Input: dimensioned drawing with shaded views. Units: mm. Origin: part minimum x, y, z. A direction names the side the tool comes from. Round coordinates to 2 decimals unless told otherwise and drop trailing zeros. Loops run counter-clockwise (first coordinate to the right, second up) from the corner with the lowest first, then second, coordinate; pieces in that order, holes last. Notation, with made-up numbers: (68.25, -16.75) - (101.25, -16.75) arc R24 cw to (101.25, 14.25) - close; hole circle Ø11 at (83, -29). An arc over 180 degrees is marked (long way). Answer as a JSON object with one key per item and string values. Group by question number.
Item 1: Line query: line 1 (X direction, y = 1.85, z = 44) (1 decimal); line 2 (Y direction, x = 10, z = 42); line 3 (Z direction, x = 35.5, y = 2.85). Output: solid intervals per line, ascending.
Item 2: Section B-B (y = 1.3). Return the cut outline in (x, z) (1 decimal), plus the area to 3 significant figures.
Item 3: Draft query along Z for the marked faces 1, 2 and 3. Return one class per face: released by +Z, released by -Z, zero draft, split by the parting line, or undercut.
Item 4: First-contact query: pin 1 (1.6 mm diameter, centred on x = 55.48, z = 19.3, fed in from +Y); pin 2 (1 mm diameter, centred on x = 50.5, y = 1.5, fed in from +Z) (1 decimal); pin 3 (1 mm diameter, centred on x = 34.5, y = 2.5, fed in from -Z) (1 decimal); pin 4 (16.5 mm diameter, centred on x = 66, z = 36.5, fed in from +Y). Flat tips, straight axial feed; report the tip coordinate or a pass-through.
Item 5: Reachability of the marked faces 4 and 5 from +Z, -Z, +X, -X, +Y, -Y: full face, straight path, thin tool, end or side. Return the list, or none.
Item 6: Section A-A (z = 41). Return the cut outline in (x, y) (1 decimal).
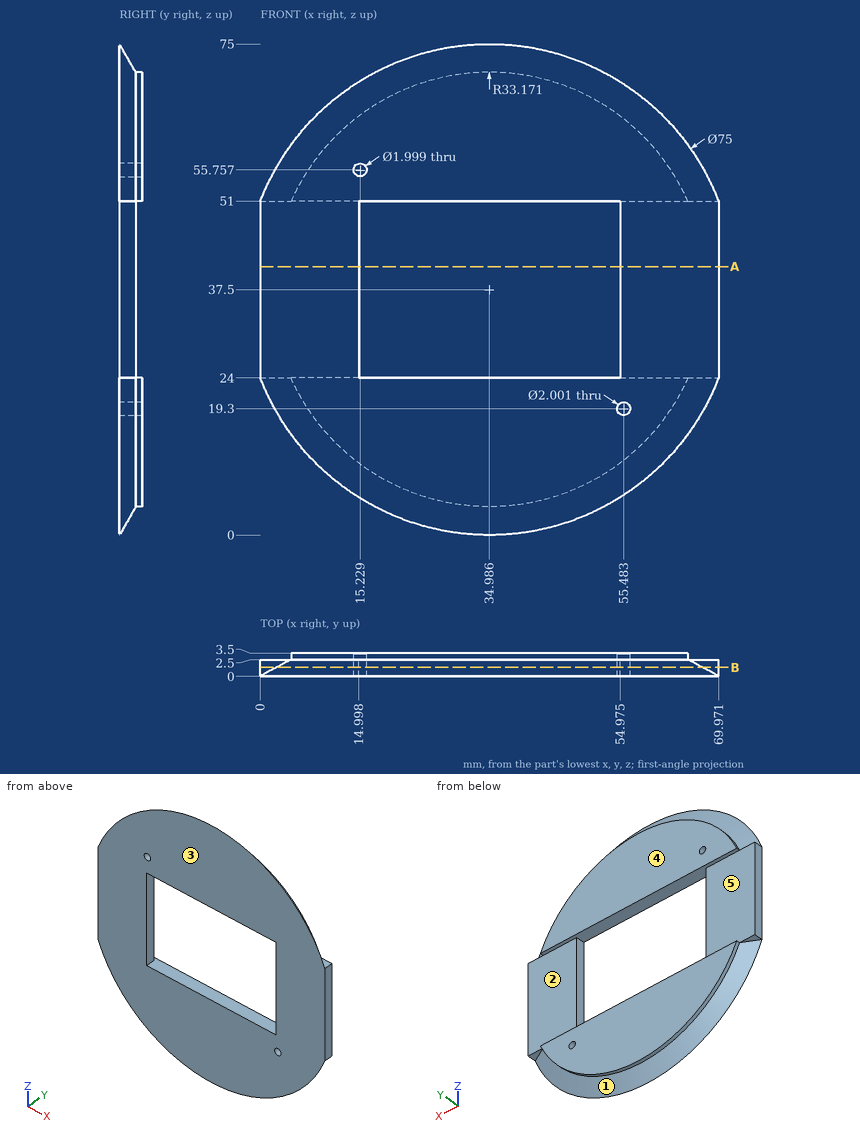
Values:
{
 "1": {"line 1": "x = 0 to 15, 55 to 70", "line 2": "y = 0 to 2.5", "line 3": "z = 4.33 to 24, 51 to 70.67"},
 "2": {"outline": "(0, 24) - (2.4, 24) arc R35.2 ccw to (67.5, 24) - (70, 24) - (70, 51) - (67.5, 51) arc R35.2 ccw to (2.4, 51) - (0, 51) - close; hole circle Ø2 at (15.2, 55.8); hole (15, 24) - (55, 24) - (55, 51) - (15, 51) - close; hole circle Ø2 at (55.5, 19.3)", "area": "2,850 mm^2"},
 "3": {"face 1": "released by -Z", "face 2": "undercut", "face 3": "zero draft"},
 "4": {"pin 1": "passes through", "pin 2": "stops at z = 69.8", "pin 3": "stops at z = 3.5", "pin 4": "stops at y = 2.5"},
 "5": {"face 4": "+Z, -Z, +X, -X, +Y", "face 5": "+X, -X, +Y"},
 "6": {"outline": "(0, 0) - (15, 0) - (15, 2.5) - (0, 2.5) - close; (55, 0) - (70, 0) - (70, 2.5) - (55, 2.5) - close"}
}
